```python
from build123d import *

# Parameters (mm, degrees)
BOSS_EXTRUDE1_DEPTH     = 34.925
F_1_4_CLEARANCE_HOLE1_D = 6.7564
F_1_4_CLEARANCE_HOLE2_D = 6.7564
CHAMFER1_SIZE           = 12.7


with BuildPart() as part:
    # Sketch1 → Boss-Extrude1 (new, symmetric)
    with BuildSketch(Plane.XY):
        Polygon((0, 38.1), (0, 0), (25.4, 0), (25.4, 6.35), (6.35, 6.35), (6.35, 38.1), align=None)
    extrude(amount=BOSS_EXTRUDE1_DEPTH, both=True)

    # 1/4 Clearance Hole1 (through all)
    with Locations(Plane.ZY):
        with Locations((-28.575, 25.4), (28.575, 25.4)):
            Hole(F_1_4_CLEARANCE_HOLE1_D / 2)

    # 1/4 Clearance Hole2 (through all)
    with Locations(Plane(origin=(0, 6.35, 0), x_dir=(1, 0, 0), z_dir=(0, 1, 0))):
        with Locations((15.875, 0)):
            Hole(F_1_4_CLEARANCE_HOLE2_D / 2)

    # Chamfer1
    chamfer1_edges = [part.edges().sort_by_distance(p)[0] for p in [
        (25.4, 3.175, 34.925),
        (25.4, 3.175, -34.925),
    ]]
    chamfer(chamfer1_edges, length=CHAMFER1_SIZE)


solid = part.part
```
Read the model definition and answer for the solid it produces. Units are mm, in the model's axes. A direction names the side the tool comes from. Give positions to 0.01 mm unless a question says otherwise; leave off trailing zeros. Loops run counter-clockwise (first coordinate to the right, second up) from the corner with the lowest first, then second, coordinate; pieces in that order, holes last.
Item 1: The part is cut by section C-C (x = 17). Write down the section's boundary in (y, z) (3 decimals).
Item 2: The part is cut by section B-B (y = 25.4). Write down the section's boundary in (x, z) (3 decimals), and give its area (3 significant figures).
Item 3: For faces 1 (the flat face through (6.35, 22, 0)), 2 (the cylindrical face through (12.754, 3.131, 1.294)), determine the directions among +Z, -Z, +X, -X, +Y, -Y from which every point of the face is accessible in a straight line to the end or side of a thin tool.
Item 4: The part is cut by section D-D (y = 5.5). Write down the section's boundary in (x, z) (3 decimals).
Item 5: The part is cut by section A-A (z = 0). Write down the section's boundary in (x, y).
Item 6: Find the intervals of material crossed by line 1 along Y through (x, z) = (1, 25.5); line 2 along Y through (x, z) = (11.75, -21), in increasing order.
Item 7: The mould has two halves that part along Z. Classify faces 3 (the flat face through (3, 38.1, 0)), 4 (the flat face through (19.139, 3.131, -28.486)), 5 (the flat face through (3, 19, 34.925)), 6 (the cylindrical face through (3.22, 22.4, 27.02)): released by +Z, released by -Z, zero draft, split by the parting line, or undercut.
Item 8: Each of these flat-tipped pins is pushed along its axis until it touches: pin 1 Ø1 at (x, z) = (16.5, 8.5) entering from +Y; pin 2 Ø9.5 at (y, z) = (26, 17.5) entering from +X. Where does it stop, or does it pass through?
Taken from the geometry:
1. outline: (0, -30.625) - (6.35, -30.625) - (6.35, -3.185) - (0, -3.185) - close; (0, 3.185) - (6.35, 3.185) - (6.35, 30.625) - (0, 30.625) - close
2. outline: (0, -34.925) - (6.35, -34.925) - (6.35, -31.953) - (0, -31.953) - close; (0, -25.197) - (6.35, -25.197) - (6.35, 25.197) - (0, 25.197) - close; (0, 31.953) - (6.35, 31.953) - (6.35, 34.925) - (0, 34.925) - close
2. area: 358 mm2
3. face 1: +Z, -Z, +X, +Y
3. face 2: +Y, -Y
4. outline: (0, -34.925) - (12.7, -34.925) - (25.4, -22.225) - (25.4, 22.225) - (12.7, 34.925) - (0, 34.925) - close; hole circle Ø6.756 at (15.875, 0)
5. outline: (0, 0) - (12.5, 0) - (12.5, 6.35) - (6.35, 6.35) - (6.35, 38.1) - (0, 38.1) - close; (19.25, 0) - (25.4, 0) - (25.4, 6.35) - (19.25, 6.35) - close
6. line 1: y = 0 to 24, 26.8 to 38.1
6. line 2: y = 0 to 6.35
7. face 3: zero draft
7. face 4: released by -Z
7. face 5: released by +Z
7. face 6: undercut
8. pin 1: stops at y = 6.35
8. pin 2: stops at x = 6.35
